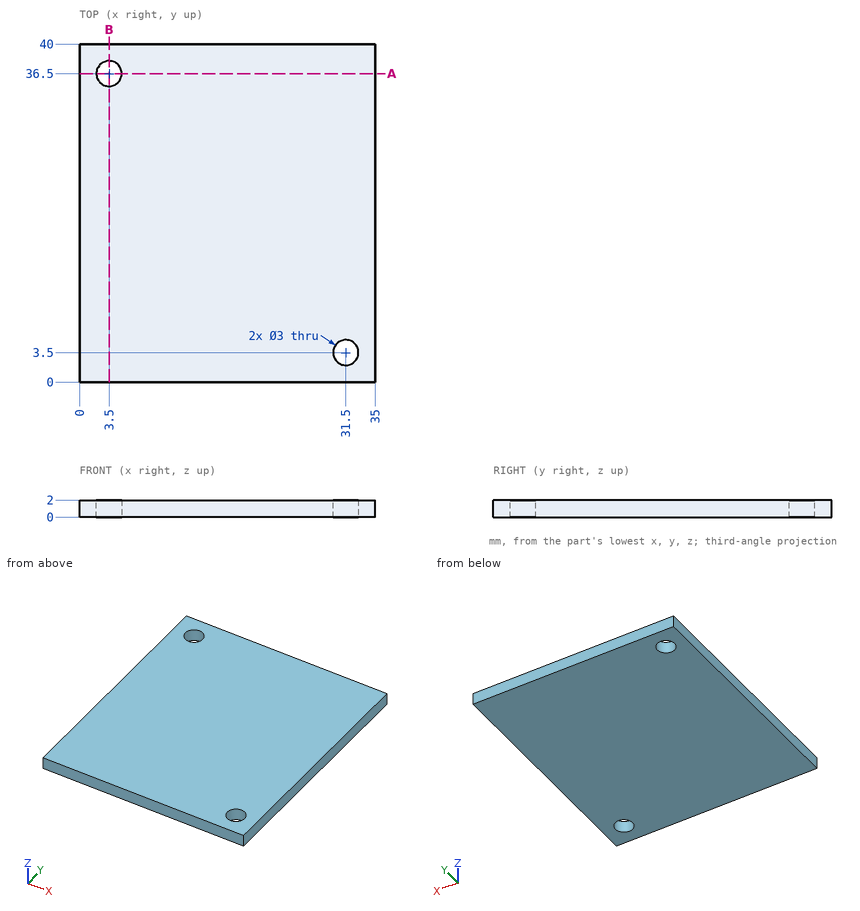
Job drawing, mm, ordinate dimensions from the low corner. One solid piece. Coordinates: 2 decimals unless noted, no trailing zeros. Order: outer loops, then holes, each group sorted by start corner. A loop starts at its lowest first (then second) coordinate and runs counter-clockwise, first axis right, second up. Notation, with made-up numbers: M -24.75,55 L -1.75,55 A17 ccw -1.75,88 Z; hole C 67.5,-3 d2. An arc over 180 degrees is marked long. Answer as CSV lines item,"result".
(1) Band-saw the part on B-B, the plane x = 3.5. List the corners of the cut face in (y, z).
Geometry says:
outline,"M 0,0 L 35,0 L 35,2 L 0,2 Z; M 38,0 L 40,0 L 40,2 L 38,2 Z"
(2) Flat gauge pin, fed straight in: pin 1 (2.5 mm diameter, centred on x = 3.5, y = 36.5, fed in from -Z). Where does the tip first touch, or does it go through?
Geometry says:
pin 1,"passes through"
(3) Band-saw the part on A-A, the plane y = 36.5. List the corners of the cut face in (x, z), then the cut area to 3 significant figures.
Geometry says:
outline,"M 0,0 L 2,0 L 2,2 L 0,2 Z; M 5,0 L 35,0 L 35,2 L 5,2 Z"
area,"64.0 mm2"
(4) Wall check: line 1 along Y through (x, z) = (31.5, 0.45); line 2 along X through (y, z) = (35.5, 0.7); line 3 along X through (y, z) = (3, 0.2). Give the ranges that are in metal, low to high.
Geometry says:
line 1,"y = 0 to 2, 5 to 40"
line 2,"x = 0 to 2.38, 4.62 to 35"
line 3,"x = 0 to 30.09, 32.91 to 35"
